```python
from build123d import *

# Parameters (mm, degrees)
F0_R     = 1.5
F1_DEPTH = 8


with BuildPart() as f1:
    # F0 (on Top) → F1 (new body)
    with BuildSketch(Plane.XY):
        with BuildLine():
            ThreePointArc((0, 7.982175), (7.982175, 0), (0, -7.982175))
            Line((0, -7.982175), (-28.84924, -7.982175))
            ThreePointArc((-28.84924, -7.982175), (30.069351, 0), (-28.84924, 7.982175))
            Line((-28.84924, 7.982175), (0, 7.982175))
        make_face()
        with Locations((-6.679961, -21.217225)):
            Circle(F0_R, mode=Mode.SUBTRACT)
        with Locations((-5.188019, 20.355852)):
            Circle(F0_R, mode=Mode.SUBTRACT)
        with Locations((20.707492, 0)):
            Circle(F0_R, mode=Mode.SUBTRACT)
    extrude(amount=F1_DEPTH)


solid = f1.part
```
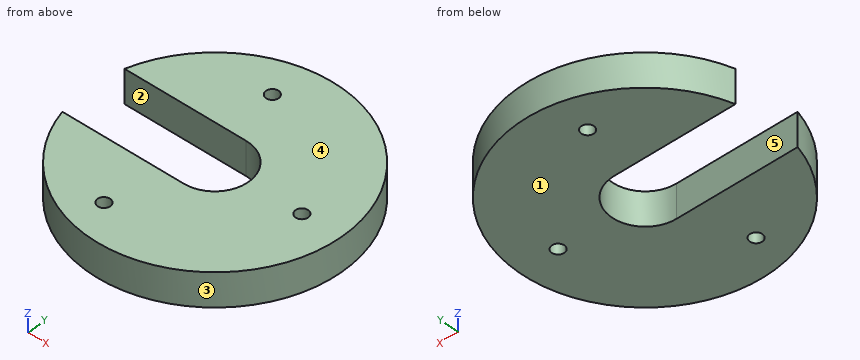
Verification items for the finished model (mm, model axes). Face numbers are marked on the shaded views. A direction names the side the tool comes from. Give positions to 0.01 mm unless a question says otherwise; leave off trailing zeros. Loops run counter-clockwise (first coordinate to the right, second up) from the corner with the lowest first, then second, coordinate; pieces in that order, holes last.
1. Section check D-D, the plane y = 26. Enter the section's corners in (x, z).
2. Set-up check for the marked faces 1 and 2: record each of +Z, -Z, +X, -X, +Y, -Y from which the full face is reachable in a straight line by a thin tool's end or side.
3. Section check C-C, the plane x = -12. Enter the section's corners in (y, z).
4. Section check A-A, the plane y = 0. Enter the section's corners in (x, z), then the cut area to 3 significant figures.
5. Section check B-B, the plane z = 4.5. Enter the section's corners in (x, y), then the cut area to 3 significant figures.
6. Mould release check, pull along Y, two halves, no side actions. Record for the marked faces 3, 4 and 5: released by +Y, released by -Y, zero draft, split by the parting line, or undercut.
7. Go/stop test with flat-tipped pins: pin 1 Ø2 at (y, z) = (-20, 7) entering from -X; pin 2 Ø4 at (x, z) = (-20.5, 2.5) entering from +Y; pin 3 Ø4 at (x, y) = (-6.68, -21.22) entering from -Z; pin 4 Ø1.5 at (x, z) = (-3.5, 4.5) entering from +Y. Record where each tip stops, or that it passes through.
8. Thickness scan on line 1 (Y direction, x = 7, z = 3.25); line 2 (Y direction, x = -12, z = 3.5); line 3 (X direction, y = -0.5, z = 6.5). Record the ranges inside material, lowest first.
Geometry says:
1. outline: (-14.9, 0) - (15.04, 0) - (15.04, 8) - (-14.9, 8) - close
2. face 1: -Z, +X, -X, +Y, -Y
2. face 2: +Z, -Z, -X
3. outline: (-27.47, 0) - (-7.98, 0) - (-7.98, 8) - (-27.47, 8) - close; (7.98, 0) - (27.47, 0) - (27.47, 8) - (7.98, 8) - close
4. outline: (7.98, 0) - (19.21, 0) - (19.21, 8) - (7.98, 8) - close; (22.21, 0) - (30.07, 0) - (30.07, 8) - (22.21, 8) - close
4. area: 153 mm2
5. outline: (-28.85, -7.98) arc R30 ccw (long way) to (-28.85, 7.98) - (0, 7.98) arc R7.98 cw to (0, -7.98) - close; hole circle Ø3 at (-6.68, -21.22); hole circle Ø3 at (-5.19, 20.36); hole circle Ø3 at (20.71, 0)
5. area: 2,230 mm2
6. face 3: split by the parting line
6. face 4: zero draft
6. face 5: undercut
7. pin 1: stops at x = -23.15
7. pin 2: stops at y = 23.56
7. pin 3: stops at z = 0
7. pin 4: stops at y = 29.87
8. line 1: y = -29.19 to -3.84, 3.84 to 29.19
8. line 2: y = -27.47 to -7.98, 7.98 to 27.47
8. line 3: x = 7.97 to 19.29, 22.12 to 30.07
